Solid Edge part; units mm, degrees
sketch "Sketch1" plane through (0, 0, 0) normal (0, 0, 1) x (1, 0, 0)
  line L0 (-2.5, 12.3) -> (-2.5, 7.5)
  line L1 (-2.5, 7.5) -> (-0.1732, 7.5)
  line L2 (-0.1732, 7.5) -> (0, 7.8)
  line L3 (0, 7.8) -> (0.1732, 7.5)
  line L4 (0.1732, 7.5) -> (2.5, 7.5)
  line L5 (2.5, 7.5) -> (2.5, 12.3)
  line L6 (2.5, 12.3) -> (2.1, 12.3)
  line L7 (2.1, 12.3) -> (2.1, 11.6)
  arc A0 (2.1, 11.6) -> (-2.1, 11.6) centre (0, 11.6) cw
  line L8 (-2.1, 11.6) -> (-2.1, 12.3)
  line L9 (-2.1, 12.3) -> (-2.5, 12.3)
revolve "RevolvedProtrusion1" add sketch "Sketch1" angle 360 about axis through (2.5, 0, 0) along (-1, 0, 0)
The model under review builds one solid part; all positions refer to its coordinate system, in mm. A direction names the side the tool comes from. Round coordinates to 2 decimals unless told otherwise and drop trailing zeros. Order: outer loops, then holes, each group sorted by start corner. A loop starts at its lowest first (then second) coordinate and runs counter-clockwise, first axis right, second up.
Item 1: Add section A-A, the plane y = 0. State the section outline as (x, z) points, and give its area (3 significant figures).
Working result:
outline: (-2.5, -12.3) - (-2.1, -12.3) - (-2.1, -11.6) arc R2.1 cw to (2.1, -11.6) - (2.1, -12.3) - (2.5, -12.3) - (2.5, -7.5) - (0.17, -7.5) - (0, -7.8) - (-0.17, -7.5) - (-2.5, -7.5) - close; (-2.5, 7.5) - (-0.17, 7.5) - (0, 7.8) - (0.17, 7.5) - (2.5, 7.5) - (2.5, 12.3) - (2.1, 12.3) - (2.1, 11.6) arc R2.1 cw to (-2.1, 11.6) - (-2.1, 12.3) - (-2.5, 12.3) - close
area: 28.2 mm2
Item 2: Machinability: for faces 5 (the flat face through (2.1, 4.5, 10.9)), 6 (the cylindrical face through (-2.3, -2.7, 12)), which of the approach directions +Z, -Z, +X, -X, +Y, -Y give a long, thin tool a straight path to every point of the face, cutting with its end or side? Answer none if there is none.
Working result:
face 5: none
face 6: +X, -X
Item 3: Add section C-C, the plane x = -1. State the section outline as (y, z) points.
Working result:
outline: circle Ø19.51 at (0, 0); hole circle Ø15 at (0, 0)
Item 4: Draft analysis for pull direction Z (two halves, no side actions). For faces 1 (the cylindrical face through (-1.32, -7.493, 0.33)), 2 (the flat face through (-2.1, 4.5, 10.9)), 3 (the cylindrical face through (1.353, -7.493, 0.33)), 4 (the cylindrical face through (2.3, -2.7, 12)), state which applies: released by +Z, released by -Z, zero draft, split by the parting line, or undercut.
Working result:
face 1: undercut
face 2: zero draft
face 3: undercut
face 4: split by the parting line
Item 5: For pin 1 (12 mm diameter, centred on y = -5, z = 3, fed in from -X), flat-tipped, find the tip position at first contact; note if it passes through.
Working result:
pin 1: stops at x = -2.5
Item 6: To check wall thickness, follow probe 1 along X at (y, z) = (7, 9.5); probe 2 along Y at (x, z) = (-1.35, 0); probe 3 along Y at (x, z) = (-0.05, 4). State the ranges of each line that lie inside material, in increasing order.
Working result:
probe 1: x = -2.5 to -2.1, 2.1 to 2.5
probe 2: y = -9.99 to -7.5, 7.5 to 9.99
probe 3: y = -8.62 to -6.6, 6.6 to 8.62
